from build123d import *

# Parameters (mm, degrees)
BOSS_EXTRUDE1_DEPTH = 13
SKETCH2_R           = 2.25
CUT_EXTRUDE1_DEPTH  = 3
SKETCH3_R           = 2
BOSS_EXTRUDE2_DEPTH = 3
BOSS_EXTRUDE3_START = 3
SKETCH4_R           = 2
BOSS_EXTRUDE3_DEPTH = 3
CUT_EXTRUDE2_DEPTH  = 3.5
CUT_EXTRUDE3_START  = -3.5
CUT_EXTRUDE3_DEPTH  = 3.5
FILLET1_R           = 6.5
FILLET2_R           = 6.5
SKETCH7_R           = 3.9
CUT_EXTRUDE4_DEPTH  = 68.830671528
CUT_EXTRUDE5_START  = -2
CUT_EXTRUDE5_DEPTH  = 2


with BuildPart() as part:
    # Sketch1 → Boss-Extrude1 (new body)
    with BuildSketch(Plane.XY):
        Polygon((3, 0), (3, 34), (36, 34), (36, 0), (39, 0), (39, 42), (35.5, 42), (35.5, 56), (3.5, 56), (3.5, 42), (0, 42), (0, 0), align=None)
    extrude(amount=BOSS_EXTRUDE1_DEPTH)

    # Sketch2 → Cut-Extrude1 (cut)
    with BuildSketch(Plane.ZY):
        with Locations((6.5, 5.293988539)):
            Circle(SKETCH2_R)
    extrude(amount=-CUT_EXTRUDE1_DEPTH, mode=Mode.SUBTRACT)

    # Sketch3 → Boss-Extrude2 (add)
    with BuildSketch(Plane.ZY.offset(-3.5)):
        with Locations(Location((6.5, 49.5, 0), (0, 0, 180))):
            Circle(SKETCH3_R)
    extrude(amount=BOSS_EXTRUDE2_DEPTH)

    # Sketch4 → Boss-Extrude3 (add)
    with BuildSketch(Plane(origin=(35.5, 0, 0), x_dir=(0, 0, -1), z_dir=(1, 0, 0)).offset(BOSS_EXTRUDE3_START)):
        with Locations((-6.5, 49.5)):
            Circle(SKETCH4_R)
    extrude(amount=-BOSS_EXTRUDE3_DEPTH)

    # Sketch5 → Cut-Extrude2 (cut)
    with BuildSketch(Plane(origin=(39, 0, 0), x_dir=(0, 0, -1), z_dir=(1, 0, 0))):
        with BuildLine():
            Line((0, 35.5), (0, 45))
            Line((0, 45), (-13, 45))
            Line((-13, 45), (-13, 35.5))
            ThreePointArc((-13, 35.5), (-6.5, 40.300735254), (0, 35.5))
        make_face()
    extrude(amount=-CUT_EXTRUDE2_DEPTH, mode=Mode.SUBTRACT)

    # Sketch6 → Cut-Extrude3 (cut)
    with BuildSketch(Plane.ZY.offset(CUT_EXTRUDE3_START)):
        with BuildLine():
            Line((13, 35.5), (13, 45))
            Line((13, 45), (0, 45))
            Line((0, 45), (0, 35.5))
            ThreePointArc((0, 35.5), (6.5, 40.300735254), (13, 35.5))
        make_face()
    extrude(amount=CUT_EXTRUDE3_DEPTH, mode=Mode.SUBTRACT)

    # Fillet1
    fillet1_edges = [part.edges().sort_by_distance(p)[0] for p in [
        (19.5, 56, 13),
        (19.5, 56, 0),
    ]]
    fillet(fillet1_edges, radius=FILLET1_R - 0.0001)  # a hair under: the kernel refuses the full size

    # Fillet2
    fillet2_edges = [part.edges().sort_by_distance(p)[0] for p in [
        (37.5, 0, 13),
        (37.5, 0, 0),
        (1.5, 0, 13),
        (1.5, 0, 0),
    ]]
    fillet(fillet2_edges, radius=FILLET2_R - 0.0001)  # a hair under: the kernel refuses the full size

    # Sketch7 → Cut-Extrude4 (cut, through all)
    with BuildSketch(Plane.ZY.offset(-36)):
        with Locations((6.5, 5.293988539)):
            Circle(SKETCH7_R)
    extrude(amount=-CUT_EXTRUDE4_DEPTH, mode=Mode.SUBTRACT)

    # Sketch8 → Cut-Extrude5 (cut)
    with BuildSketch(Plane(origin=(39, 0, 0), x_dir=(0, 0, -1), z_dir=(1, 0, 0)).offset(CUT_EXTRUDE5_START)):
        with BuildLine():
            Line((-8.989087294, 20.527321872), (-10.382976178, 5.657988539))
            ThreePointArc((-10.382976178, 5.657988539), (-6.5, 1.393988539), (-2.617023822, 5.657988539))
            Line((-2.617023822, 5.657988539), (-4.010912706, 20.527321872))
            ThreePointArc((-4.010912706, 20.527321872), (-6.5, 22.793988539), (-8.989087294, 20.527321872))
        make_face()
    extrude(amount=CUT_EXTRUDE5_DEPTH, mode=Mode.SUBTRACT)


solid = part.part
For this review, take the finished solid that the model builds, in its own axes (mm). A direction names the side the tool comes from. Coordinates: 2 decimals unless noted, no trailing zeros. Loops run counter-clockwise (first coordinate to the right, second up) from the corner with the lowest first, then second, coordinate; pieces in that order, holes last. Notation, with made-up numbers: (13.25, 5.25) - (58.25, 5.25) arc R6 ccw to (58.25, 14.25) - close; hole circle Ø4 at (-1, -28). An arc over 180 degrees is marked (long way). Use a Markdown table: item, result. Add a question column.
Item 1: We need section D-D (z = 1). Give the boundary of the cut face in (x, y).
Item 2: We need section A-A (y = 30). Give the boundary of the cut face in (x, z).
Item 3: Mouldability with a two-part tool opening along Z and no side actions: class faces 1 (the face through (37.521, 1.955, 1.854)), 2 (the face through (2.021, 51.452, 6.934)), 3 (the face through (37.146, 1.487, 5.655)), 4 (the face through (0.5, 49, 7)) as pulls with the +Z half, pulls with the -Z half, needs draft (parallel to the pull), parting line crosses it, or undercut.
Item 4: Tool access review of faces 5 (the face through (38.5, 50, 7)), 6 (the face through (37.986, 13.197, 9.676)), 7 (the face through (3.5, 46, 6)), 8 (the face through (36, 17, 6)): name each direction out of +Z, -Z, +X, -X, +Y, -Y from which nothing blocks a thin tool from reaching the whole face with its end or side.
Item 5: For line 1 (Y direction, x = 1.25, z = 6.5); line 2 (Y direction, x = 37.5, z = 6.5); line 3 (X direction, y = 29, z = 11.5), list the stretches that pass through material, from the lowest coordinate up.
Item 6: We need section B-B (z = 7.75). Give the number of separate pieces and of enclosed holes in the cut face, and give its area (3 significant figures).
Item 7: Insertion check: pin 1 Ø1.2 at (y, z) = (50.5, 6) entering from -X; pin 2 Ø10 at (x, y) = (12, 25) entering from -Z; pin 3 Ø4 at (y, z) = (44, 7) entering from -X; pin 4 Ø3 at (x, z) = (19, 4) entering from -Y. Each pin has a flat end and moves straight along its axis. Give the tip position at first contact, or say it passes through.
Results list:
| question | item | result |
|---|---|---|
| 1 | outline | (0, 3.04) - (3, 3.04) - (3, 34) - (36, 34) - (36, 3.04) - (39, 3.04) - (39, 37.5) - (35.5, 37.5) - (35.5, 52.96) - (3.5, 52.96) - (3.5, 37.5) - (0, 37.5) - close |
| 2 | outline | (0, 0) - (3, 0) - (3, 13) - (0, 13) - close; (36, 0) - (39, 0) - (39, 13) - (36, 13) - close |
| 3 | face 1 | pulls with the -Z half |
| 3 | face 2 | parting line crosses it |
| 3 | face 3 | undercut |
| 3 | face 4 | needs draft |
| 4 | face 5 | +Z, -Z, +X, +Y |
| 4 | face 6 | +X |
| 4 | face 7 | -X |
| 4 | face 8 | +Z, -Z, -Y |
| 5 | line 1 | y = 0 to 3.04, 7.54 to 40.3, 47.5 to 51.5 |
| 5 | line 2 | y = 0 to 1.39, 22.79 to 40.3, 47.5 to 51.5 |
| 5 | line 3 | x = 0 to 3, 36 to 39 |
| 6 | separate pieces | 3 |
| 6 | enclosed holes | 0 |
| 6 | area | 905 mm^2 |
| 7 | pin 1 | stops at x = 0.5 |
| 7 | pin 2 | passes through |
| 7 | pin 3 | stops at x = 3.5 |
| 7 | pin 4 | stops at y = 34 |
